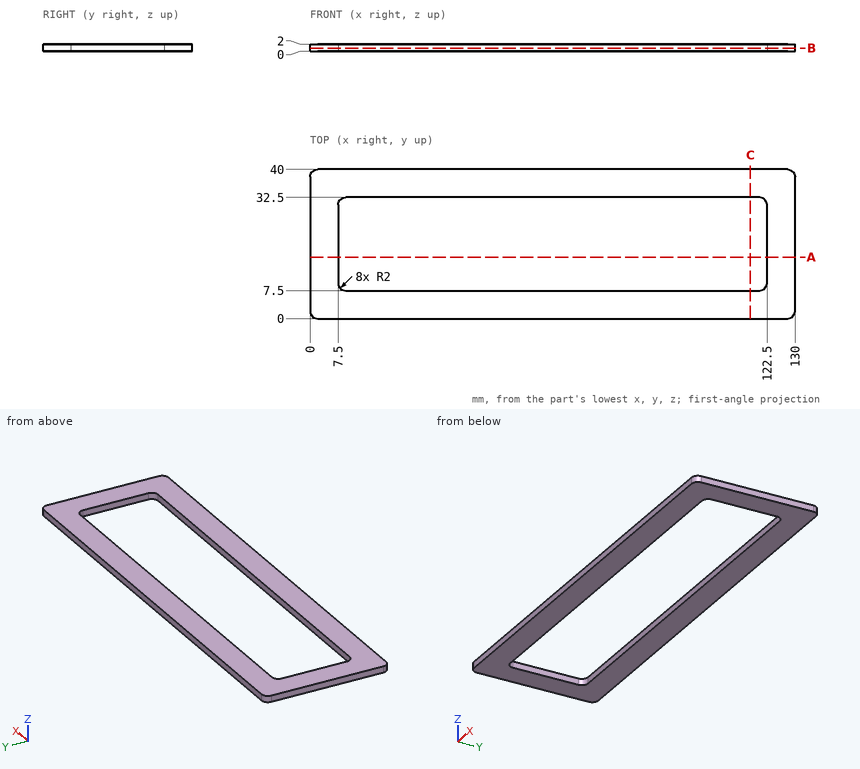
Could you check a few things on this drawing? It's one solid part, dimensions in mm from its lowest x, y, z. Give positions to 0.01 mm unless a question says otherwise; leave off trailing zeros. Order: outer loops, then holes, each group sorted by start corner. A loop starts at its lowest first (then second) coordinate and runs counter-clockwise, first axis right, second up. Notation, with made-up numbers: (-9.5, 81) - (16.5, 81) arc R25 cw to (16.5, 99) - close; hole circle Ø5 at (26, 88). An arc over 180 degrees is marked (long way). Answer as a JSON object with one key per item and string values. Group by question number.
Item 1: If we section it at B-B on z = 0.9: Please give me the cut outline in (x, y), and give its area (4 significant figures).
Item 2: Please list where these lines run through material, in increasing order: probe 1 along Y at (x, z) = (37, 0.7); probe 2 along X at (y, z) = (15.5, 1.4); probe 3 along Y at (x, z) = (9, 1.7).
Item 3: If we section it at A-A on y = 16.5: Please give me the cut outline in (x, z).
Item 4: For P1, Ø0.6, axis at y = 16.5, z = 0.5, coming from the -X side, with a flat end and sliding along its axis, tell me the tip position at first contact or that it passes through.
Item 5: If we section it at C-C on x = 118: Please give me the cut outline in (y, z).
Result set:
{
 "1": {"outline": "(0, 2) arc R2 ccw to (2, 0) - (128, 0) arc R2 ccw to (130, 2) - (130, 38) arc R2 ccw to (128, 40) - (2, 40) arc R2 ccw to (0, 38) - close; hole (7.5, 9.5) arc R2 ccw to (9.5, 7.5) - (120.5, 7.5) arc R2 ccw to (122.5, 9.5) - (122.5, 30.5) arc R2 ccw to (120.5, 32.5) - (9.5, 32.5) arc R2 ccw to (7.5, 30.5) - close", "area": "2,325 mm²"},
 "2": {"probe 1": "0 to 7.5, 32.5 to 40", "probe 2": "0 to 7.5, 122.5 to 130", "probe 3": "0 to 7.56, 32.44 to 40"},
 "3": {"outline": "(0, 0) - (7.5, 0) - (7.5, 2) - (0, 2) - close; (122.5, 0) - (130, 0) - (130, 2) - (122.5, 2) - close"},
 "4": {"P1": "x = 0"},
 "5": {"outline": "(0, 0) - (7.5, 0) - (7.5, 2) - (0, 2) - close; (32.5, 0) - (40, 0) - (40, 2) - (32.5, 2) - close"}
}
